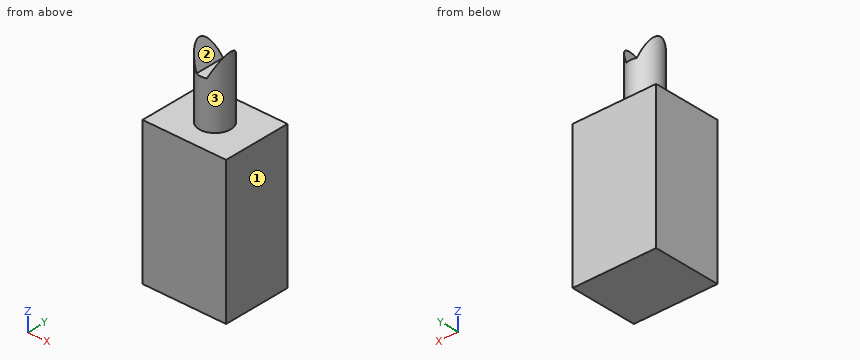
from build123d import *

# Parameters (mm, degrees)
F0_W     = 32
F0_H     = 26
F1_DEPTH = 55
F2_R     = 6
F3_DEPTH = 26
F5_DEPTH = 25


with BuildPart() as f1:
    # F0 (on Top) → F1 (new body)
    with BuildSketch(Plane.XY):
        with Locations((16, 13)):
            Rectangle(F0_W, F0_H)
    extrude(amount=F1_DEPTH)

    # F2 (on face) → F3 (join)
    with BuildSketch(Plane.XY.offset(55)):
        with Locations((16, 13)):
            Circle(F2_R)
    extrude(amount=F3_DEPTH)

    # F4 (on face) → F5 (cut)
    with BuildSketch(Plane.XZ):
        Polygon((22, 81), (10, 81), (14, 73), (18, 73), align=None)
    extrude(amount=-F5_DEPTH, mode=Mode.SUBTRACT)


solid = f1.part
Geometry check sheet. Reference: the model listing, model coordinates, mm. Face numbers are marked on the shaded views. Coordinates: 2 decimals unless noted, no trailing zeros. Loops run counter-clockwise (first coordinate to the right, second up) from the corner with the lowest first, then second, coordinate; pieces in that order, holes last. Notation, with made-up numbers: (67.5, 63) - (72.5, 63) arc R15 ccw to (72.5, 73) - close; hole circle Ø1 at (16, 36). An arc over 180 degrees is marked (long way). Use one line per item in the form item = value. Start each with the question number.
Item 1: Section check C-C, the plane z = 62.5. Enter the section's corners in (x, y), and give its area (3 significant figures).
Item 2: Section check A-A, the plane x = 16. Enter the section's corners in (y, z).
Item 3: Mould release check, pull along X, two halves, no side actions. Record for the marked faces 1, 2 and 3: +X half, -X half, draft (parallel to the pull), parting line (faces both ways), or undercut.
Item 4: Section check D-D, the plane y = 17.75. Enter the section's corners in (x, z).
Item 5: Gauge pin test, flat ends, axial feed: pin 1 (3 mm diameter, centred on x = 16, y = 11, fed in from +Z); pin 2 (1.5 mm diameter, centred on x = 8.5, z = 67.5, fed in from -Y); pin 3 (4 mm diameter, centred on x = 3.5, y = 13.5, fed in from +Z). Record the tip position at first contact, or that the pin passes through.
Item 6: Section check B-B, the plane y = 13. Enter the section's corners in (x, z), and give its area (3 significant figures).
Item 7: Thickness scan on probe 1 along Z at (x, y) = (8, 9.5); probe 2 along Z at (x, y) = (16.5, 10.5); probe 3 along X at (y, z) = (9.25, 66.5). Record the ranges inside material, lowest first.
Computed:
q1.outline = circle Ø12 at (16, 13)
q1.area = 113 mm2
q2.outline = (0, 0) - (26, 0) - (26, 55) - (19, 55) - (19, 73) - (7, 73) - (7, 55) - (0, 55) - close
q3.face_1 = +X half
q3.face_2 = undercut
q3.face_3 = parting line
q4.outline = (0, 0) - (32, 0) - (32, 55) - (19.67, 55) - (19.67, 76.33) - (18, 73) - (14, 73) - (12.33, 76.33) - (12.33, 55) - (0, 55) - close
q5.pin_1 = 73
q5.pin_2 = through
q5.pin_3 = 55
q6.outline = (0, 0) - (32, 0) - (32, 55) - (22, 55) - (22, 81) - (18, 73) - (14, 73) - (10, 81) - (10, 55) - (0, 55) - close
q6.area = 2,010 mm2
q7.probe_1 = 0 to 55
q7.probe_2 = 0 to 73
q7.probe_3 = 11.32 to 20.68
